Build history of the part. All positions in model axes, mm. Give positions to 0.01 mm unless a question says otherwise; leave off trailing zeros. Order: outer loops, then holes, each group sorted by start corner. A loop starts at its lowest first (then second) coordinate and runs counter-clockwise, first axis right, second up. Notation, with made-up numbers: (-6, 51) -> (10, 51) arc R17 cw to (10, 77) -> close; hole circle Ø11 at (8.25, -25). An arc over 180 degrees is marked (long way). Use a Markdown table: item, result. Add a question column.
```python
from build123d import *

# Parameters (mm, degrees)
F1_DEPTH = 0.635


with BuildPart() as f1:
    # F0 (on Front) → F1 (new body, symmetric)
    with BuildSketch(Plane.XZ):
        with BuildLine():
            Line((-50.8, -6.35), (50.8, -6.35))
            Line((50.8, -6.35), (50.8, -3.175))
            ThreePointArc((50.8, -3.175), (47.625, 0), (50.8, 3.175))
            Line((50.8, 3.175), (50.8, 6.35))
            Line((50.8, 6.35), (-50.8, 6.35))
            Line((-50.8, 6.35), (-50.8, 3.175))
            ThreePointArc((-50.8, 3.175), (-48.554936, 2.245064), (-47.625, 0))
            ThreePointArc((-47.625, 0), (-48.554936, -2.245064), (-50.8, -3.175))
            Line((-50.8, -3.175), (-50.8, -6.35))
        make_face()
        with BuildLine():
            Line((50.8, -3.175), (50.8, -6.35))
            ThreePointArc((50.8, -6.35), (57.15, 0), (50.8, 6.35))
            Line((50.8, 6.35), (50.8, 3.175))
            ThreePointArc((50.8, 3.175), (53.045064, 2.245064), (53.975, 0))
            ThreePointArc((53.975, 0), (53.045064, -2.245064), (50.8, -3.175))
        make_face()
        with BuildLine():
            ThreePointArc((-50.8, 6.35), (-57.15, 0), (-50.8, -6.35))
            Line((-50.8, -6.35), (-50.8, -3.175))
            ThreePointArc((-50.8, -3.175), (-53.975, 0), (-50.8, 3.175))
            Line((-50.8, 3.175), (-50.8, 6.35))
        make_face()
    extrude(amount=F1_DEPTH, both=True)


solid = f1.part
```
(1) Band-saw the part on B-B on z = -5.25. Give the cut face in (x, y) (3 decimals), plus the area to 3 significant figures.
(2) Wall check: probe 1 along X at (y, z) = (-0.25, 1); probe 2 along X at (y, z) = (-0.2, -1.25); probe 3 along Z at (x, y) = (50.5, -0.5). Give the ranges that are in metal, low to high.
(3) Band-saw the part on A-A on y = -0.3. Give the cut face in (x, z) (3 decimals).
Response:
| question | item | result |
|---|---|---|
| 1 | outline | (-54.372, -0.635) -> (54.372, -0.635) -> (54.372, 0.635) -> (-54.372, 0.635) -> close |
| 1 | area | 138 mm² |
| 2 | probe 1 | x = -57.07 to -53.81, -47.79 to 47.79, 53.81 to 57.07 |
| 2 | probe 2 | x = -57.03 to -53.72, -47.88 to 47.88, 53.72 to 57.03 |
| 2 | probe 3 | z = -6.35 to -3.16, 3.16 to 6.35 |
| 3 | outline | (-50.8, -6.35) -> (50.8, -6.35) arc R6.35 ccw to (50.8, 6.35) -> (-50.8, 6.35) arc R6.35 ccw to start; hole circle Ø6.35 at (-50.8, 0); hole circle Ø6.35 at (50.8, 0) |
